```python
from build123d import *

# Parameters (mm, degrees)
BOSS_EXTRUDE1_DEPTH = 20
CUT_EXTRUDE1_DEPTH  = 130.325171564
HOLE1_D             = 10
CHAMFER1_SIZE       = 8


with BuildPart() as part:
    # Sketch1 → Boss-Extrude1 (new, symmetric)
    with BuildSketch(Plane.XY):
        Polygon((-70, 0), (-70, 15), (-40, 15), (-40, 65), (-15, 65), (-15, 42), (15, 42), (15, 65), (40, 65), (40, 15), (70, 15), (70, 0), (15, 0), (15, 25), (-15, 25), (-15, 0), align=None)
    extrude(amount=BOSS_EXTRUDE1_DEPTH, both=True)

    # Sketch2 → Cut-Extrude1 (cut, through all)
    with BuildSketch(Plane.ZY.offset(40)):
        with BuildLine():
            Line((-20, 65), (-20, 45))
            ThreePointArc((-20, 45), (-14.142135624, 59.142135624), (0, 65))
            Line((0, 65), (-20, 65))
        make_face()
    cut_extrude1 = extrude(amount=-CUT_EXTRUDE1_DEPTH, mode=Mode.SUBTRACT)

    # Mirror1: Cut-Extrude1 across plane
    add(cut_extrude1.mirror(Plane.XY), mode=Mode.SUBTRACT)

    # Hole1 (through all)
    with Locations(Plane(origin=(40, 0, 0), x_dir=(0, 0, -1), z_dir=(1, 0, 0))):
        with Locations((0, 50)):
            Hole(HOLE1_D / 2)

    # Chamfer1
    chamfer1_edges = [part.edges().sort_by_distance(p)[0] for p in [
        (70, 7.5, 20),
        (-70, 7.5, 20),
    ]]
    chamfer(chamfer1_edges, length=CHAMFER1_SIZE)


solid = part.part
```
CAD build for the part. Positions are in the model's coordinates, mm. A direction names the side the tool comes from. Give positions to 0.01 mm unless a question says otherwise; leave off trailing zeros. Loops run counter-clockwise (first coordinate to the right, second up) from the corner with the lowest first, then second, coordinate; pieces in that order, holes last. Notation, with made-up numbers: M 20,74 L 58,74 A27 ccw 58,98 Z; hole C -23.75,32.5 d4. An arc over 180 degrees is marked long. Use one line per item in the form item = value.
Item 1: Slice it at B-B (x = -21.5). List the corners of the cut face in (y, z).
Determined:
outline = M 0,-20 L 45,-20 A20 ccw 45,20 L 0,20 Z; hole C 50,0 d10
Item 2: Slice it at A-A (y = 16.5). List the corners of the cut face in (x, z), plus the area to 3 significant figures.
Determined:
outline = M -40,-20 L -15,-20 L -15,20 L -40,20 Z; M 15,-20 L 40,-20 L 40,20 L 15,20 Z
area = 2,000 mm2
Item 3: Which spindle directions (+Z, -Z, +X, -X, +Y, -Y) get a long thin tool onto all of the face, cutting with end or side? Do faces 5 (the face through (-40, 40, 0)), 6 (the face through (15, 56, 0)), 7 (the face through (40, 40, 0)). Say none if no direction does.
Determined:
face_5 = +Z, -Z, -X, +Y
face_6 = +Z, -Z, +Y
face_7 = +Z, -Z, +X, +Y
Item 4: Slice it at D-D (y = 57). List the corners of the cut face in (x, z).
Determined:
outline = M -40,-16 L -15,-16 L -15,16 L -40,16 Z; M 15,-16 L 40,-16 L 40,16 L 15,16 Z
Item 5: Two-plate mould, pull along Z, no slides. Class faces 1 (the face through (1, 28, -20)), 2 (the face through (-70, 7, -4)), 3 (the face through (66, 8, 16)), 4 (the face through (27.325, 54.957, -0.651)): pulls with the +Z half, pulls with the -Z half, needs draft (parallel to the pull), parting line crosses it, or undercut.
Determined:
face_1 = pulls with the -Z half
face_2 = needs draft
face_3 = pulls with the +Z half
face_4 = undercut
Item 6: Flat gauge pins, fed straight in: pin 1 (9 mm diameter, centred on x = 3, z = -1, fed in from +Y); pin 2 (8 mm diameter, centred on y = 50, z = 0, fed in from -X); pin 3 (9 mm diameter, centred on x = -60, z = 0, fed in from +Y); pin 4 (18.5 mm diameter, centred on y = 58, z = -7.5, fed in from -X). Where does each tip first touch, or does it go through?
Determined:
pin_1 = 42
pin_2 = through
pin_3 = 15
pin_4 = -40
Item 7: Slice it at C-C (y = 50). List the corners of the cut face in (x, z).
Determined:
outline = M -40,-19.36 L -15,-19.36 L -15,-5 L -40,-5 Z; M -40,5 L -15,5 L -15,19.36 L -40,19.36 Z; M 15,-19.36 L 40,-19.36 L 40,-5 L 15,-5 Z; M 15,5 L 40,5 L 40,19.36 L 15,19.36 Z
Item 8: Drill centre lines: probe 1 along X at (y, z) = (49, 18.5); probe 2 along X at (y, z) = (13.5, -5); probe 3 along Y at (x, z) = (-31.5, 0). Where is each one in solid material? Low to high. Write a range as from..to.
Determined:
probe_1 = -40..-15, 15..40
probe_2 = -70..-15, 15..70
probe_3 = 0..45, 55..65
